Source: CAD feature listing. Evaluate the final solid. Frame: model axes, mm. A direction names the side the tool comes from. Round coordinates to 2 decimals unless told otherwise and drop trailing zeros. Loops run counter-clockwise (first coordinate to the right, second up) from the corner with the lowest first, then second, coordinate; pieces in that order, holes last.
Item 1: Section query A-A on y = 4. Return loops of the section in (x, z).
Item 2: Section query D-D on y = -97. Return loops of the section in (x, z), then the cut area to 3 significant figures.
Item 3: Section query C-C on x = 29. Return loops of the section in (y, z), then the cut area to 3 significant figures.
Item 4: Pull-direction query (X, two-part tool) for faces 3 (the cylindrical face through (87.08, -97.86, 186.48)), 4 (the flat face through (39, -48, 188)); classes: released by +X, released by -X, zero draft, split by the parting line, or undercut.
Item 5: Access query for faces 1 (the cylindrical face through (-42.15, -69.99, 186.52)), 2 (the flat face through (39, -48, 185)). Directions: +Z, -Z, +X, -X, +Y, -Y. A direction counts if a zero-diameter tool reaches every point of the face in a straight line with its end or side. Return the directions, or none.
Item 6: Section query B-B on z = 186.55. Return loops of the section in (x, y).
Item 7: First-contact query: P1, Ø1.5, axis at y = -8, z = 186, coming from the -X side; P2, Ø3.5, axis at x = -85, y = -97, coming from the +Z side. Flat tips, straight axial feed; report the tip coordinate or a pass-through.
Item 8: Ray query, L1, parallel to Y at x = 85, z = 187.3; L2, parallel to Y at x = -32, z = 186; L3, parallel to Y at x = 14, z = 185.9. Return the intervals inside material, ascending.
```python
from build123d import *

# Parameters (mm, degrees)
SKETCH259_R          = 2.25
SKETCH259_R_2        = 1.5
PAD029_DEPTH         = 3
POCKET019_DEPTH      = 0.001
POCKET019_DEPTH_BACK = 3.001
POCKET020_DEPTH      = 5


with BuildPart() as part:
    # Sketch259 → Pad029 (new body)
    with BuildSketch(Plane.XY):
        Polygon((91, 90), (-40, 90), (-40, -63), (-91, -63), (-91, -103), (91, -103), align=None)
        with Locations((85, 85)):
            Circle(SKETCH259_R, mode=Mode.SUBTRACT)
        with Locations((85, -97)):
            Circle(SKETCH259_R, mode=Mode.SUBTRACT)
        with Locations((-85, -97)):
            Circle(SKETCH259_R, mode=Mode.SUBTRACT)
        with Locations((-31, 84)):
            Circle(SKETCH259_R_2, mode=Mode.SUBTRACT)
    extrude(amount=PAD029_DEPTH)

    # Sketch258 → Pocket019 (cut, two sides)
    with BuildSketch(Plane.XY) as pocket019_sk:
        with BuildLine():
            ThreePointArc((13.5, 56.497619), (14, -48.5), (14.5, 56.497619))
            Line((13.5, 56.497619), (14.5, 56.497619))
        make_face()
    extrude(amount=-POCKET019_DEPTH, mode=Mode.SUBTRACT)
    extrude(pocket019_sk.sketch, amount=POCKET019_DEPTH_BACK, mode=Mode.SUBTRACT)

    # Sketch260 → Pocket020 (cut)
    with BuildSketch(Plane.XY.offset(3)):
        with BuildLine():
            ThreePointArc((-55, -63), (-49.142136, -77.142136), (-35, -83))
            Line((0, -83), (-35, -83))
            Line((0, -73), (0, -83))
            Line((-35, -73), (0, -73))
            ThreePointArc((-45, -63), (-42.071068, -70.071068), (-35, -73))
            Line((-55, -63), (-45, -63))
        make_face()
    extrude(amount=-POCKET020_DEPTH, mode=Mode.SUBTRACT)


with BuildPart() as part_1:
    # Body013 placement: moved
    add(part.part.moved(Location((0, 0, 185))))


solid = part_1.part
```
Data:
1. outline: (-40, 185) - (-38.5, 185) - (-38.5, 188) - (-40, 188) - close; (66.5, 185) - (91, 185) - (91, 188) - (66.5, 188) - close
2. outline: (-91, 185) - (-87.25, 185) - (-87.25, 188) - (-91, 188) - close; (-82.75, 185) - (82.75, 185) - (82.75, 188) - (-82.75, 188) - close; (87.25, 185) - (91, 185) - (91, 188) - (87.25, 188) - close
2. area: 519 mm2
3. outline: (-103, 185) - (-46.31, 185) - (-46.31, 188) - (-103, 188) - close; (54.31, 185) - (90, 185) - (90, 188) - (54.31, 188) - close
3. area: 277 mm2
4. face 3: undercut
4. face 4: zero draft
5. face 1: +Z, -Z
5. face 2: -Z, +X, -X, +Y, -Y
6. outline: (-91, -103) - (91, -103) - (91, 90) - (-40, 90) - (-40, -63) - (-45, -63) arc R10 ccw to (-35, -73) - (0, -73) - (0, -83) - (-35, -83) arc R20 cw to (-55, -63) - (-91, -63) - close; hole circle Ø4.5 at (-85, -97); hole circle Ø3 at (-31, 84); hole (13.5, 56.5) arc R52.5 ccw (long way) to (14.5, 56.5) - close; hole circle Ø4.5 at (85, -97); hole circle Ø4.5 at (85, 85)
7. P1: stops at x = -40
7. P2: passes through
8. L1: y = -103 to -99.25, -94.75 to 82.75, 87.25 to 90
8. L2: y = -103 to -83, -73 to -21.3, 29.3 to 82.88, 85.12 to 90
8. L3: y = -103 to -48.5, 56.5 to 90
